Autodesk Inventor part; units mm, degrees
ref_plane "Work Plane1" through (20, 0, 0) normal (1, 0, 0) x (0, 1, 0)
ref_plane "XZ Plane" through (0, 0, 0) normal (0, 1, 0) x (-1, 0, 0)
ref_plane "XY Plane" through (0, 0, 0) normal (0, 0, 1) x (1, 0, 0)
ref_plane "Work Plane1" through (20, 0, 0) normal (1, 0, 0) x (0, 1, 0)
sketch "Sketch7" plane through (0, 0, 0) normal (1, 0, 0) x (0, 1, 0)
  circle A0 centre (0, 0) radius 7.5
  circle A1 centre (0, 0) radius 20
  dimension "d28" = 15
  dimension "d29" = 40
extrude "Wheel" add sketch "Sketch7" along normal blind 18
sketch "Sketch8" plane through (0, 0, 0) normal (1, 0, 0) x (0, 1, 0)
  circle A0 centre (0, 0) radius 8.5
  circle A1 centre (0, 0) radius 13.5
  dimension "d32" = 17
  dimension "d33" = 27
extrude "Extrusion7" cut sketch "Sketch8" along normal blind 17
sketch "Sketch9" plane through (0, 0, 0) normal (-1, 0, 0) x (0, 0, 1)
  circle A0 centre (0, 0) radius 11.0642
extrude "Extrusion8" cut sketch "Sketch9" against normal blind 3
fillet "Fillet1" radius 2 1 edges at (0, -20, 0)
fillet "Fillet2" radius 1 1 edges at (0, -13.5, 0)
shell "Shell1" thickness 1.5 removed faces 1 at (18, 15.6396, -1.5954)
sketch "Sketch10" plane through (18, 0, 0) normal (1, 0, 0) x (0, 0, -1)
  circle A0 centre (0, 0) radius 8.5
  circle A1 centre (0, 0) radius 7.5
  dimension "d41" = 17
extrude "Extrusion9" add sketch "Sketch10" along normal blind 8
sketch "Sketch11" plane through (0, 0, 0) normal (0, 0, 1) x (1, 0, 0)
  line L0 (26, -8.5) -> (26, 8.5)
  line L1 (18, 8.5) -> (18, -8.5)
  line L2 (26, 7.5) -> (26, -7.5)
  line L3 (26, -5) -> (23, -5)
  line L4 (23, -5) -> (23, 5)
  line L5 (23, 5) -> (26, 5)
  line L6 (26, 5) -> (26, -5)
  line L7 (0, 0) -> (9.4673, 0) construction
  dimension "d44" = 3
  dimension "d45" = 10
  dimension "d46" = 5
extrude "Extrusion10" cut sketch "Sketch11" against normal blind 20
equation "\"d46\" = 0.5 * d45"
properties part number "RearWheelLeft"
Read the model definition and answer for the solid it produces. Units are mm, in the model's axes. A direction names the side the tool comes from. Give positions to 0.01 mm unless a question says otherwise; leave off trailing zeros. Write each loop counter-clockwise with the first axis right and the second up, starting at its lowest first coordinate (ties: lowest second). Pieces come first, ordered by that corner, then holes. Notation, with made-up numbers: M 27,83 L 69,83 A29 ccw 69,103 Z; hole C -26.5,36.25 d9. An arc over 180 degrees is marked long. One line per item, written item: value. Start each with the question number.
(1) Flat-ended cylindrical pins translate along their axes: pin 1 Ø3 at (y, z) = (-2, -6.5) entering from +X; pin 2 Ø1.5 at (x, y) = (16, 10) entering from +Z; pin 3 Ø21.5 at (y, z) = (3, -1.5) entering from -X; pin 4 Ø12 at (y, z) = (0, 0) entering from +X. Find the tip coordinate at first contact, or state that the pin passes through.
(2) Determine the mould class of faces 1 (the flat face through (0, 1, 15)), 2 (the cylindrical face through (9.902, 4.57, -7.167)), 3 (the cylindrical face through (21.94, -0.37, 8.49)) for opening direction Z: pulls with the +Z half, pulls with the -Z half, needs draft (parallel to the pull), parting line crosses it, or undercut.
(3) Find the intervals of material crossed by line 1 (Z direction, x = 5.75, y = 0); line 2 (Z direction, x = 7, y = -1); line 3 (Z direction, x = 16.5, y = -11), in increasing order.
(4) Find section B-B (x = 22). Determine the outline of the cut face in (y, z), plus the area to 3 significant figures.
(5) A tool of negligible diameter and unlimited length cuts with its end or side. For faces 4 (the flat face through (3, -8, 0)), 5 (the flat face through (24, 5, -6)), 6 (the cylindrical face through (9.888, -4.336, 19.524)), 7 (the flat face through (18, 6.5, -6.5)), from which of +Z, -Z, +X, -X, +Y, -Y can it reach the whole face along a straight path? Write none if from no direction.
(6) Find section A-A (x = 10.25). Determine the outline of the cut face in (y, z).
Results below:
1. pin 1: stops at x = 23
1. pin 2: stops at z = 17.73
1. pin 3: stops at x = 0.08
1. pin 4: passes through
2. face 1: needs draft
2. face 2: undercut
2. face 3: parting line crosses it
3. line 1: z = -20 to -18.5, -15 to -13.5, -8.5 to -7.5, 7.5 to 8.5, 13.5 to 15, 18.5 to 20
3. line 2: z = -19.97 to -18.47, -14.97 to -13.46, -8.44 to -7.43, 7.43 to 8.44, 13.46 to 14.97, 18.47 to 19.97
3. line 3: z = -16.7 to -14.87, -10.2 to -7.83, 7.83 to 10.2, 14.87 to 16.7
4. outline: C 0,0 d17; hole C 0,0 d15
4. area: 50.3 mm^2
5. face 4: -X
5. face 5: -Z, +X
5. face 6: +X, -X
5. face 7: +X
6. outline: C 0,0 d40; C 0,0 d30; C 0,0 d17; hole C 0,0 d37; hole C 0,0 d27; hole C 0,0 d15
